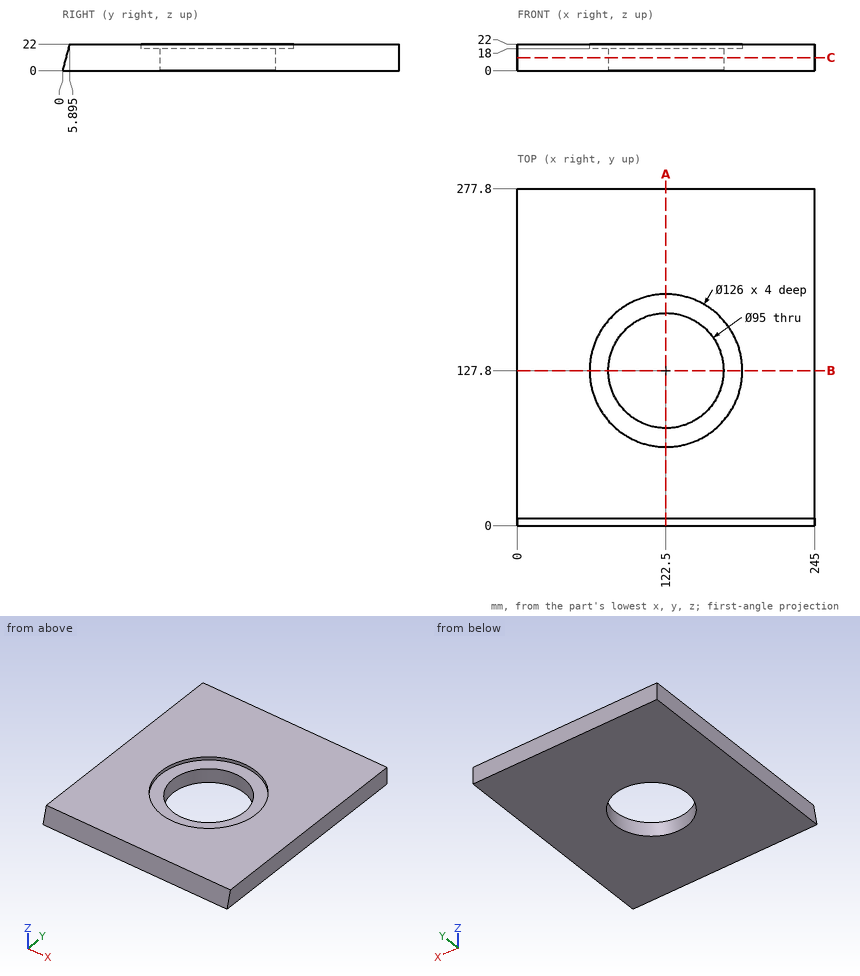
Geometry check sheet. Reference: drawing and pictorial views, mm from the part's lowest x, y, z. Coordinates: 2 decimals unless noted, no trailing zeros. Order: outer loops, then holes, each group sorted by start corner. A loop starts at its lowest first (then second) coordinate and runs counter-clockwise, first axis right, second up. Notation, with made-up numbers: (-24.75, 85.25) -> (10.25, 85.25) arc R22 cw to (10.25, 106.25) -> close; hole circle Ø8 at (78.25, 53.5). An arc over 180 degrees is marked (long way). Write item = value, one per line. Start each with the question number.
1) Cross-section at B-B (y = 127.8). Enter the section's corners in (x, z).
2) Cross-section at A-A (x = 122.5). Enter the section's corners in (y, z) (3 decimals).
3) Cross-section at C-C (z = 10.75). Enter the section's corners in (x, y), then the cut area to 3 significant figures.
4) Material ranges on L1, parallel to X at y = 125.5, z = 20.5; L2, parallel to Z at x = 155, y = 163.5; L3, parallel to Y at x = 122.5, z = 5.25, recorded low to high.
Ans:
q1.outline = (0, 0) -> (75, 0) -> (75, 18) -> (59.5, 18) -> (59.5, 22) -> (0, 22) -> close; (170, 0) -> (245, 0) -> (245, 22) -> (185.5, 22) -> (185.5, 18) -> (170, 18) -> close
q2.outline = (0, 0) -> (80.3, 0) -> (80.3, 18) -> (64.8, 18) -> (64.8, 22) -> (5.895, 22) -> close; (175.3, 0) -> (277.8, 0) -> (277.8, 22) -> (190.8, 22) -> (190.8, 18) -> (175.3, 18) -> close
q3.outline = (0, 2.88) -> (245, 2.88) -> (245, 277.8) -> (0, 277.8) -> close; hole circle Ø95 at (122.5, 127.8)
q3.area = 60,300 mm²
q4.L1 = 0 to 59.54, 185.46 to 245
q4.L2 = 0 to 18
q4.L3 = 1.41 to 80.3, 175.3 to 277.8
